Part print with two shaded views. Sizes in mm from the minimum x, y, z corner. Round coordinates to 2 decimals unless told otherwise and drop trailing zeros. Loops run counter-clockwise (first coordinate to the right, second up) from the corner with the lowest first, then second, coordinate; pieces in that order, holes last. Notation, with made-up numbers: (67.5, 60) -> (110.5, 60) arc R33 ccw to (110.5, 98) -> close; hole circle Ø11 at (35.25, 4.5). An arc over 180 degrees is marked (long way). Answer as a JSON object with one key per item and string values. Group by question number.
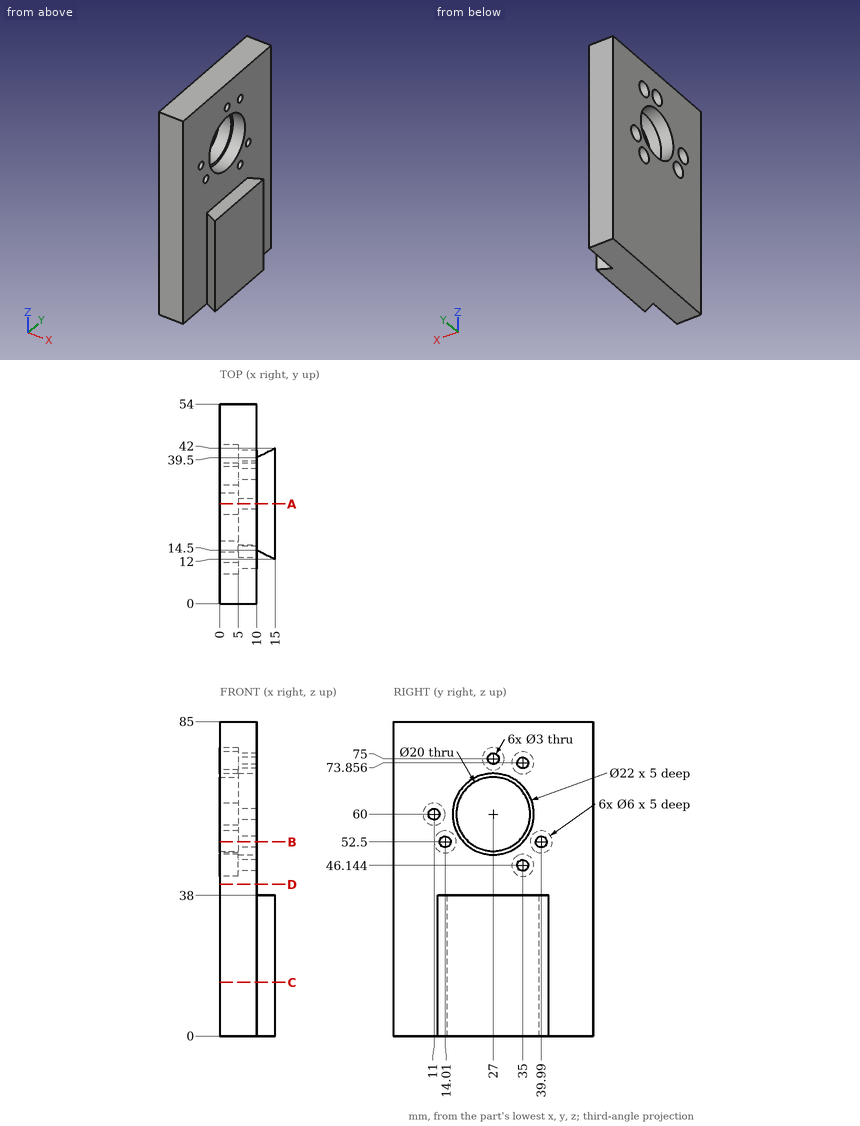
Item 1: Band-saw the part on B-B, the plane z = 52.5. List the corners of the cut face in (x, y) (1 decimal).
Item 2: Band-saw the part on A-A, the plane y = 27. List the corners of the cut face in (x, z), plus the area to 3 significant figures.
Item 3: Band-saw the part on C-C, the plane z = 14.5. List the corners of the cut face in (x, y).
Item 4: Drill centre lines: line 1 (Y direction, x = 3.75, z = 52.5) (1 decimal); line 2 (Z direction, x = 1.25, y = 13) (1 decimal); line 3 (X direction, y = 49.5, z = 26). Where is each one in solid material? Low to high.
Item 5: Band-saw the part on D-D, the plane z = 41. List the corners of the cut face in (x, y).
Item 6: Drop flat-ended pins along their axis: pin 1 Ø7 at (y, z) = (35, 46.14) entering from +X; pin 2 Ø13 at (y, z) = (27, 60) entering from -X; pin 3 Ø8 at (y, z) = (43.5, 15) entering from +X; pin 4 Ø4 at (y, z) = (27, 75) entering from -X. Give the stop position or say it passes through.
Entries:
{
 "1": {"outline": "(0, 0) -> (10, 0) -> (10, 12.5) -> (5, 12.5) -> (5, 11) -> (0, 11) -> close; (0, 17) -> (5, 17) -> (5, 15.5) -> (10, 15.5) -> (10, 19) -> (5, 19) -> (5, 20.4) -> (0, 20.4) -> close; (0, 33.6) -> (5, 33.6) -> (5, 35) -> (10, 35) -> (10, 38.5) -> (5, 38.5) -> (5, 37) -> (0, 37) -> close; (0, 43) -> (5, 43) -> (5, 41.5) -> (10, 41.5) -> (10, 54) -> (0, 54) -> close"},
 "2": {"outline": "(0, 0) -> (15, 0) -> (15, 38) -> (10, 38) -> (10, 49) -> (5, 49) -> (5, 50) -> (0, 50) -> close; (0, 70) -> (5, 70) -> (5, 71) -> (10, 71) -> (10, 73.5) -> (5, 73.5) -> (5, 72) -> (0, 72) -> close; (0, 78) -> (5, 78) -> (5, 76.5) -> (10, 76.5) -> (10, 85) -> (0, 85) -> close", "area": "785 mm²"},
 "3": {"outline": "(0, 0) -> (10, 0) -> (10, 14.5) -> (15, 12) -> (15, 42) -> (10, 39.5) -> (10, 54) -> (0, 54) -> close"},
 "4": {"line 1": "0 to 11, 17 to 20.4, 33.6 to 37, 43 to 54", "line 2": "0 to 49.7, 55.3 to 57.8, 62.2 to 85", "line 3": "0 to 10"},
 "5": {"outline": "(0, 0) -> (10, 0) -> (10, 54) -> (0, 54) -> close"},
 "6": {"pin 1": "x = 10", "pin 2": "through", "pin 3": "x = 15", "pin 4": "x = 5"}
}
